```python
from build123d import *

# Parameters (mm, degrees)
BOSS_EXTRUDE1_DEPTH = 4
SKETCH2_R           = 1.6
CUT_EXTRUDE1_DEPTH  = 5
SKETCH3_R           = 5
BOSS_EXTRUDE2_DEPTH = 6
SKETCH5_R           = 1.6
CUT_EXTRUDE2_DEPTH  = 6


with BuildPart() as part:
    # Sketch1 → Boss-Extrude1 (new body)
    with BuildSketch(Plane(origin=(0, 0, 0), x_dir=(1, 0, 0), z_dir=(0, 1, 0))):
        with BuildLine():
            Line((0, 5), (55, 5))
            ThreePointArc((55, 5), (60, 0), (55, -5))
            Line((55, -5), (0, -5))
            ThreePointArc((0, -5), (-5, 0), (0, 5))
        make_face()
    extrude(amount=BOSS_EXTRUDE1_DEPTH)

    # Sketch2 → Cut-Extrude1 (cut, through all)
    with BuildSketch(Plane(origin=(0, 4, 0), x_dir=(1, 0, 0), z_dir=(0, 1, 0))):
        Circle(SKETCH2_R)
        with Locations((27.5, 0)):
            Circle(SKETCH2_R)
        with Locations((55, 0)):
            Circle(SKETCH2_R)
    extrude(amount=-CUT_EXTRUDE1_DEPTH, mode=Mode.SUBTRACT)

    # Sketch3 → Boss-Extrude2 (add)
    with BuildSketch(Plane.XZ):
        Circle(SKETCH3_R)
    extrude(amount=BOSS_EXTRUDE2_DEPTH)

    # Sketch5 → Cut-Extrude2 (cut)
    with BuildSketch(Plane.XZ.offset(6)):
        Circle(SKETCH5_R)
    extrude(amount=-CUT_EXTRUDE2_DEPTH, mode=Mode.SUBTRACT)


solid = part.part
```
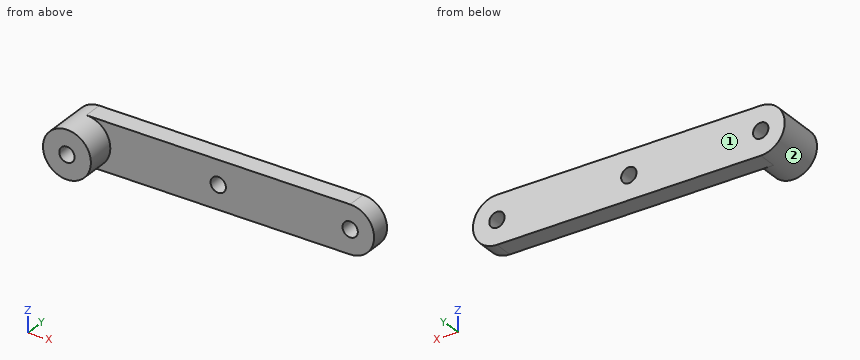
Verification items for the finished model (mm, model axes). Face numbers are marked on the shaded views. A direction names the side the tool comes from. Give positions to 0.01 mm unless a question says otherwise; leave off trailing zeros. Write each loop counter-clockwise with the first axis right and the second up, starting at its lowest first coordinate (ties: lowest second). Pieces come first, ordered by that corner, then holes. Notation, with made-up numbers: (6.5, -16) - (27.5, -16) arc R22 ccw to (27.5, 2) - close; hole circle Ø4 at (-16, 17.25). An arc over 180 degrees is marked (long way). Put each result on its own line as item: value.
Q1. Set-up check for the marked faces 1 and 2: record each of +Z, -Z, +X, -X, +Y, -Y from which the full face is reachable in a straight line by a thin tool's end or side.
Result:
face 1: +Z, -Z, +X, -X, +Y
face 2: -Y
Q2. Section check C-C on y = -3.75. Record the cut outline in (x, z), and give its area (3 significant figures).
Result:
outline: circle Ø10 at (0, 0); hole circle Ø3.2 at (0, 0)
area: 70.5 mm2
Q3. Depth check by flat-ended pin: P1, Ø1, axis at y = 0, z = -3.5, coming from the -X side; P2, Ø5, axis at x = 36, z = -2, coming from the -Y side; P3, Ø1, axis at y = -1, z = 2, coming from the +X side. Enter the tip coordinate at first touch or a pass-through.
Result:
P1: x = -4
P2: y = 0
P3: x = 4.77
Q4. Scan lines: probe 1 along X at (y, z) = (0.95, 0); probe 2 along X at (y, z) = (-1, 0). Record each from-to range of solid material in increasing order. Write a range as from..to.
Result:
probe 1: -5..-1.6, 1.6..25.9, 29.1..53.4, 56.6..60
probe 2: -5..-1.6, 1.6..5
Q5. Section check B-B on x = 27.5. Record the cut outline in (y, z), and give its area (3 significant figures).
Result:
outline: (0, -5) - (4, -5) - (4, -1.6) - (0, -1.6) - close; (0, 1.6) - (4, 1.6) - (4, 5) - (0, 5) - close
area: 27.2 mm2
Q6. Section check A-A on z = 0. Record the cut outline in (x, y), and give its area (3 significant figures).
Result:
outline: (-5, -6) - (-1.6, -6) - (-1.6, 4) - (-5, 4) - close; (1.6, -6) - (5, -6) - (5, 0) - (25.9, 0) - (25.9, 4) - (1.6, 4) - close; (29.1, 0) - (53.4, 0) - (53.4, 4) - (29.1, 4) - close; (56.6, 0) - (60, 0) - (60, 4) - (56.6, 4) - close
area: 262 mm2
Q7. Section check D-D on z = -4. Record the cut outline in (x, y), and give its area (3 significant figures).
Result:
outline: (-3, -6) - (3, -6) - (3, 0) - (58, 0) - (58, 4) - (-3, 4) - close
area: 280 mm2
